from build123d import *

# Parameters (mm, degrees)
CROQUIS2_W              = 730
CROQUIS2_H              = 330
SALIENTE_EXTRUIR2_DEPTH = 5
CROQUIS4_W              = 660
CROQUIS4_H              = 280
CORTAR_EXTRUIR1_DEPTH   = 5
SALIENTE_EXTRUIR3_DEPTH = 5


with BuildPart() as part:
    # Croquis2 → Saliente-Extruir2 (new body)
    with BuildSketch(Plane.XY):
        Rectangle(CROQUIS2_W, CROQUIS2_H)
    extrude(amount=SALIENTE_EXTRUIR2_DEPTH)

    # Croquis4 → Cortar-Extruir1 (cut)
    with BuildSketch(Plane.XY.offset(5)):
        with Locations((0, 15)):
            Rectangle(CROQUIS4_W, CROQUIS4_H)
    extrude(amount=-CORTAR_EXTRUIR1_DEPTH, mode=Mode.SUBTRACT)

    # Croquis5 → Saliente-Extruir3 (add)
    with BuildSketch(Plane.XY.offset(5)):
        Polygon((-215, -165), (-225, -165), (-225, -205), (-105, -205), (-105, -165), (-115, -165), (-115, -195), (-215, -195), align=None)
    extrude(amount=-SALIENTE_EXTRUIR3_DEPTH)


solid = part.part
Input: part model. Units: mm. Frame: model coordinates. Give positions to 0.01 mm unless a question says otherwise; leave off trailing zeros. Order: outer loops, then holes, each group sorted by start corner. A loop starts at its lowest first (then second) coordinate and runs counter-clockwise, first axis right, second up.
Q1. Ray query, probe 1 along Y at (x, z) = (-204.5, 2.8); probe 2 along X at (y, z) = (133, 3.5); probe 3 along Y at (x, z) = (-256, 2.1). Return the intervals inside material, ascending.
Checked values:
probe 1: y = -205 to -195, -165 to -125, 155 to 165
probe 2: x = -365 to -330, 330 to 365
probe 3: y = -165 to -125, 155 to 165
Q2. Section B-B on x = -157. Output: boundary loops of the cut face in (y, z).
Checked values:
outline: (-205, 0) - (-195, 0) - (-195, 5) - (-205, 5) - close; (-165, 0) - (-125, 0) - (-125, 5) - (-165, 5) - close; (155, 0) - (165, 0) - (165, 5) - (155, 5) - close
Q3. Section D-D on x = 92. Output: boundary loops of the cut face in (y, z), and give its area (3 significant figures).
Checked values:
outline: (-165, 0) - (-125, 0) - (-125, 5) - (-165, 5) - close; (155, 0) - (165, 0) - (165, 5) - (155, 5) - close
area: 250 mm2
Q4. Section C-C on z = 1. Output: boundary loops of the cut face in (x, y).
Checked values:
outline: (-365, -165) - (-225, -165) - (-225, -205) - (-105, -205) - (-105, -165) - (365, -165) - (365, 165) - (-365, 165) - close; hole (-330, -125) - (330, -125) - (330, 155) - (-330, 155) - close; hole (-215, -195) - (-115, -195) - (-115, -165) - (-215, -165) - close
Q5. Section A-A on y = 135.5. Output: boundary loops of the cut face in (x, z), and give its area (3 significant figures).
Checked values:
outline: (-365, 0) - (-330, 0) - (-330, 5) - (-365, 5) - close; (330, 0) - (365, 0) - (365, 5) - (330, 5) - close
area: 350 mm2
Q6. Contact query for flat-ended pins moving along their axis: pin 1 Ø1.5 at (y, z) = (-180.5, 2) entering from +X; pin 2 Ø2.5 at (x, z) = (-286, 3.5) entering from -Y. Output: stop coordinate, or through.
Checked values:
pin 1: stops at x = -105
pin 2: stops at y = -165
